For this review, take the finished solid that the model builds, in its own axes (mm). Face numbers are marked on the shaded views. Coordinates: 2 decimals unless noted, no trailing zeros. Loops run counter-clockwise (first coordinate to the right, second up) from the corner with the lowest first, then second, coordinate; pieces in that order, holes last. Notation, with made-up numbers: M -12,-31 L -5,-31 A17 cw -5,-22 Z; hole C 83.5,42 d7. An arc over 180 degrees is marked long. Put each result on its own line as item: value.
```python
from build123d import *

# Parameters (mm, degrees)
SKETCH_1_R          = 5.5
SKETCH_1_R_2        = 4.1
EXTRUDE_1_DEPTH     = 25
SKETCH_2_R          = 5.5
SKETCH_2_R_2        = 4
EXTRUDE_2_DEPTH     = 20
SKETCH_4_R          = 4.1
CUT_EXTRUDE_1_DEPTH = 20
CUT_EXTRUDE_START   = -20
SKETCH_5_R          = 4
CUT_EXTRUDE_2_DEPTH = 20


with BuildPart() as part:
    # 草图1 → 凸台-拉伸1 (new body)
    with BuildSketch(Plane(origin=(0, 0, 0), x_dir=(1, 0, 0), z_dir=(0, 1, 0))):
        with Locations(Location((0, 0, 0), (0, 0, 270))):
            Circle(SKETCH_1_R)
        with Locations(Location((0, 0, 0), (0, 0, 270))):
            Circle(SKETCH_1_R_2, mode=Mode.SUBTRACT)
    extrude(amount=EXTRUDE_1_DEPTH)

    # 草图2 → 凸台-拉伸2 (add)
    with BuildSketch(Plane.XY):
        with Locations((0, 5.5)):
            Circle(SKETCH_2_R)
        with Locations(Location((0, 5.5, 0), (0, 0, 180))):
            Circle(SKETCH_2_R_2, mode=Mode.SUBTRACT)
    extrude(amount=EXTRUDE_2_DEPTH)

    # 草图4 → 切除-拉伸1 (cut)
    with BuildSketch(Plane(origin=(0, 0, 0), x_dir=(1, 0, 0), z_dir=(0, 1, 0))):
        with Locations(Location((0, 0, 0), (0, 0, 270))):
            Circle(SKETCH_4_R)
    extrude(amount=CUT_EXTRUDE_1_DEPTH, mode=Mode.SUBTRACT)

    # 草图5 → 切除-拉伸2 (cut)
    with BuildSketch(Plane.XY.offset(20).offset(CUT_EXTRUDE_START)):
        with Locations((0, 5.5)):
            Circle(SKETCH_5_R)
    extrude(amount=CUT_EXTRUDE_2_DEPTH, mode=Mode.SUBTRACT)


solid = part.part
```
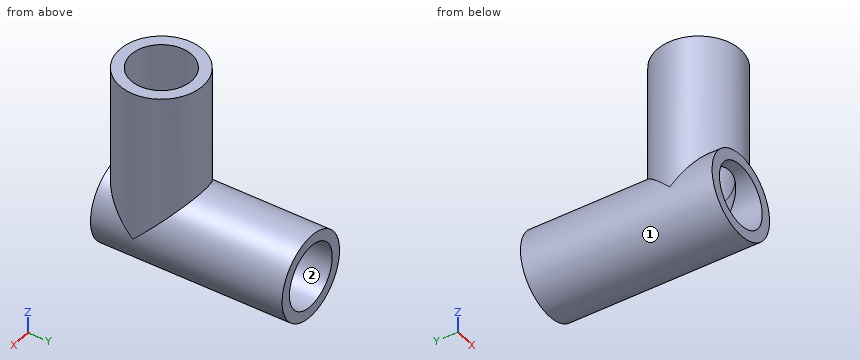
(1) Wall thickness on line 1 along Y through (x, z) = (0, 10); line 2 along Y through (x, z) = (3.25, 11.75); line 3 along X through (y, z) = (2.25, -3.75): over which ranges is each line inside the solid? List them lowest first. Write a range as [from, to].
Determined:
line 1: y = [0, 1.5], [9.5, 11]
line 2: y = [1.06, 3.17], [7.83, 9.94]
line 3: x = [-4.02, -1.66], [1.66, 4.02]
(2) Add section C-C (y = 17). Write out the cut boundary in (x, z).
Determined:
outline: C 0,0 d11; hole C 0,0 d8.2
(3) Add section B-B (z = -2.75). Write out the cut boundary in (x, y).
Determined:
outline: M -4.76,0 L -3.04,0 L -3.04,25 L -4.76,25 Z; M 3.04,0 L 4.76,0 L 4.76,25 L 3.04,25 Z
(4) Draft analysis for pull direction X (two halves, no side actions). For the marked faces 1 and 2, state which applies: +X half, -X half, draft (parallel to the pull), parting line (faces both ways), or undercut.
Determined:
face 1: parting line
face 2: undercut
(5) Add section A-A (x = -3). Write out the cut boundary in (y, z).
Determined:
outline: M 0,-4.61 L 25,-4.61 L 25,-2.79 L 0,-2.79 Z; M 0,2.79 L 2.85,2.79 L 2.85,20 L 0.89,20 L 0.89,4.61 L 0,4.61 Z; M 8.15,2.79 L 25,2.79 L 25,4.61 L 10.11,4.61 L 10.11,20 L 8.15,20 Z
(6) Add section D-D (y = 2.25). Write out the cut boundary in (x, z).
Determined:
outline: M -4.44,3.25 A5.5 ccw long 4.44,3.25 L 4.44,20 L 2.33,20 L 2.33,3.37 A4.1 cw long -2.33,3.37 L -2.33,20 L -4.44,20 Z
(7) For pin 1 (8 mm diameter, centred on y = 21.5, z = 11.5, fed in from -X) (3 decimals); pin 2 (2 mm diameter, centred on x = 4, z = 7.5, fed in from -Y), all flat-tipped, find the tip position at first contact; note any pin that passes through.
Determined:
pin 1: passes through
pin 2: stops at y = 0.89
